Check sheet for the modelled part. Datum: model origin and axes. Units: mm. A direction names the side the tool comes from. Give positions to 0.01 mm unless a question says otherwise; leave off trailing zeros. Write each loop counter-clockwise with the first axis right and the second up, starting at its lowest first coordinate (ties: lowest second). Pieces come first, ordered by that corner, then holes. Notation, with made-up numbers: M -9,-26 L 19,-26 A33 cw 19,12 Z; hole C 34.5,-35 d10. An arc over 180 degrees is marked long. Use CSV: the item, a comma, the result in double quotes. Start each with the question number.
1. Cross-section at C-C, the plane y = -9.75. Enter the section's corners in (x, z), and give its area (3 significant figures).
2. Scan lines: line 1 (Y direction, x = -31, z = 1) (3 decimals); line 2 (X direction, y = -9.5, z = 1.3); line 3 (X direction, y = 5.5, z = 1.5). Record each from-to range of solid material in increasing order.
3. Cross-section at B-B, the plane x = 31. Enter the section's corners in (y, z) (3 decimals).
4. Cross-section at A-A, the plane z = 2.4. Enter the section's corners in (x, y) (3 decimals).
5. Mould release check, pull along X, two halves, no side actions. Record for faces 1 (the face through (0, -8.5, 1)), 2 (the face through (-1, -1, 3)), 3 (the face through (-37.5, 0, 1)): +X half, -X half, draft (parallel to the pull), parting line (faces both ways), or undercut.
6. Cross-section at D-D, the plane y = 3.5. Enter the section's corners in (x, z) (3 decimals).
7. Access from +Z, -Z, +X, -X, +Y, -Y to the whole of each face (thin tool, end or side, straight path). Record for faces 4 (the face through (-1.25, -10, 2)), 5 (the face through (5, -11.5, 1)), 6 (the face through (-33.423, 3.607, 1.521)), 7 (the face through (-24, -8.5, 1)), 8 (the face through (9.25, -10, 2)).
8. Depth check by flat-ended pin: P1, Ø0.8, axis at x = -0.5, z = 1.5, coming from the -Y side; P2, Ø1.5, axis at y = -10, z = 1.5, coming from the +X side; P3, Ø4, axis at x = 31, y = 3.5, coming from the +Z side; P4, Ø0.9, axis at y = -10, z = 1.5, coming from the -X side. Enter the tip coordinate at first touch or a pass-through.
from build123d import *

# Parameters (mm, degrees)
SKETCH1_W           = 75
SKETCH1_H           = 17
BOSS_EXTRUDE1_DEPTH = 3
SKETCH2_W           = 8
SKETCH2_H           = 3
BOSS_EXTRUDE2_DEPTH = 3
SKETCH3_R           = 2.425
CUT_EXTRUDE1_DEPTH  = 3


with BuildPart() as part:
    # Sketch1 → Boss-Extrude1 (new body)
    with BuildSketch(Plane.XY):
        Rectangle(SKETCH1_W, SKETCH1_H)
    extrude(amount=BOSS_EXTRUDE1_DEPTH)

    # Sketch2 → Boss-Extrude2 (add)
    with BuildSketch(Plane(origin=(0, -8.5, 0), x_dir=(-1, 0, 0), z_dir=(0, -1, 0))):
        with Locations((5.25, -1.5)):
            Rectangle(SKETCH2_W, SKETCH2_H)
        with Locations((-5.25, -1.5)):
            Rectangle(SKETCH2_W, SKETCH2_H)
    extrude(amount=BOSS_EXTRUDE2_DEPTH)

    # Sketch3 → Cut-Extrude1 (cut)
    with BuildSketch(Plane.XY.offset(3)):
        with Locations((-31, 3.5)):
            Circle(SKETCH3_R)
        with Locations((-22.5, 3.5)):
            Circle(SKETCH3_R)
        with Locations((22.5, 3.5)):
            Circle(SKETCH3_R)
        with Locations((31, 3.5)):
            Circle(SKETCH3_R)
    extrude(amount=-CUT_EXTRUDE1_DEPTH, mode=Mode.SUBTRACT)


solid = part.part
Worked answers:
1,outline,"M -9.25,0 L -1.25,0 L -1.25,3 L -9.25,3 Z; M 1.25,0 L 9.25,0 L 9.25,3 L 1.25,3 Z"
1,area,"48.0 mm^2"
2,line 1,"y = -8.5 to 1.075, 5.925 to 8.5"
2,line 2,"x = -9.25 to -1.25, 1.25 to 9.25"
2,line 3,"x = -37.5 to -32.37, -29.63 to -23.87, -21.13 to 21.13, 23.87 to 29.63, 32.37 to 37.5"
3,outline,"M -8.5,0 L 1.075,0 L 1.075,3 L -8.5,3 Z; M 5.925,0 L 8.5,0 L 8.5,3 L 5.925,3 Z"
4,outline,"M -37.5,-8.5 L -9.25,-8.5 L -9.25,-11.5 L -1.25,-11.5 L -1.25,-8.5 L 1.25,-8.5 L 1.25,-11.5 L 9.25,-11.5 L 9.25,-8.5 L 37.5,-8.5 L 37.5,8.5 L -37.5,8.5 Z; hole C -31,3.5 d4.85; hole C -22.5,3.5 d4.85; hole C 22.5,3.5 d4.85; hole C 31,3.5 d4.85"
5,face 1,"undercut"
5,face 2,"draft"
5,face 3,"-X half"
6,outline,"M -37.5,0 L -33.425,0 L -33.425,3 L -37.5,3 Z; M -28.575,0 L -24.925,0 L -24.925,3 L -28.575,3 Z; M -20.075,0 L 20.075,0 L 20.075,3 L -20.075,3 Z; M 24.925,0 L 28.575,0 L 28.575,3 L 24.925,3 Z; M 33.425,0 L 37.5,0 L 37.5,3 L 33.425,3 Z"
7,face 4,"+Z, -Z, -Y"
7,face 5,"+Z, -Z, +X, -X, -Y"
7,face 6,"+Z, -Z"
7,face 7,"+Z, -Z, -X, -Y"
7,face 8,"+Z, -Z, +X, -Y"
8,P1,"stops at y = -8.5"
8,P2,"stops at x = 9.25"
8,P3,"passes through"
8,P4,"stops at x = -9.25"
